Design review of the part built by this model. Coordinates are the model's own, in mm. Face numbers are marked on the shaded views. A direction names the side the tool comes from. Round coordinates to 2 decimals unless told otherwise and drop trailing zeros. Loops run counter-clockwise (first coordinate to the right, second up) from the corner with the lowest first, then second, coordinate; pieces in that order, holes last. Notation, with made-up numbers: (-16.75, 10) -> (-5.75, 10) arc R26 ccw to (-5.75, 32) -> close; hole circle Ø6 at (38, -12.75). An arc over 180 degrees is marked (long way). Write each question's results on one line, items separated by ' | '. Start each with the question number.
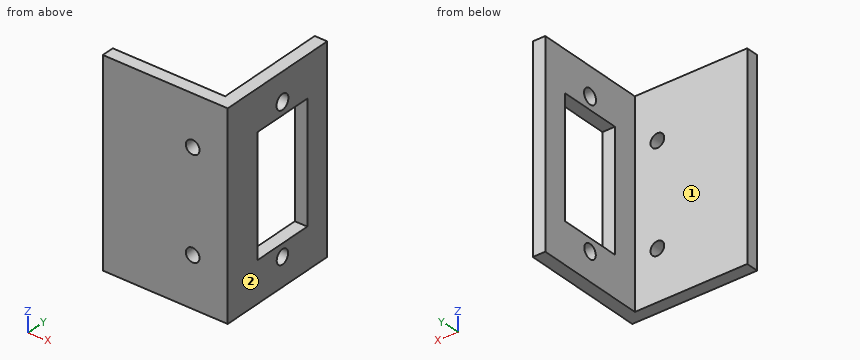
from build123d import *

# Parameters (mm, degrees)
EXTRUDE_1_DEPTH     = 16
SKETCH_4_R          = 1.15
SKETCH_4_R_2        = 1.2
SKETCH_4_W          = 19
SKETCH_4_H          = 10
CUT_EXTRUDE_1_DEPTH = 30
SKETCH_5_R          = 1.1
CUT_EXTRUDE_2_DEPTH = 30


with BuildPart() as part:
    # 草图2 → 凸台-拉伸1 (new body, symmetric)
    with BuildSketch(Plane.XY):
        Polygon((-20, 0), (0, 0), (0, 20), (-2, 20), (-2, 2), (-20, 2), align=None)
    extrude(amount=EXTRUDE_1_DEPTH, both=True)

    # 草图4 → 切除-拉伸1 (cut)
    with BuildSketch(Plane(origin=(0, 0, 0), x_dir=(0, 0, -1), z_dir=(1, 0, 0))):
        with Locations((11.5, 11)):
            Circle(SKETCH_4_R)
        with Locations((-11.5, 11)):
            Circle(SKETCH_4_R_2)
        with Locations((0, 11)):
            Rectangle(SKETCH_4_W, SKETCH_4_H)
    extrude(amount=-CUT_EXTRUDE_1_DEPTH, mode=Mode.SUBTRACT)

    # 草图5 → 切除-拉伸2 (cut)
    with BuildSketch(Plane(origin=(0, 2, 0), x_dir=(1, 0, 0), z_dir=(0, 1, 0))):
        with Locations((-5.609756098, 8)):
            Circle(SKETCH_5_R)
        with Locations((-5.609756098, -8)):
            Circle(SKETCH_5_R)
    extrude(amount=-CUT_EXTRUDE_2_DEPTH, mode=Mode.SUBTRACT)


solid = part.part
1) Insertion check: pin 1 (5.5 mm diameter, centred on x = -13.5, z = -4.5, fed in from +Y); pin 2 (5 mm diameter, centred on x = -17.5, z = 12, fed in from -Y); pin 3 (2 mm diameter, centred on y = 12.5, z = -9, fed in from -X). Each pin has a flat end and moves straight along its axis. Give the tip position at first contact, or say it passes through.
2) To check wall thickness, follow line 1 (X direction, y = 1.5, z = 8); line 2 (Y direction, x = -0.5, z = -11.5); line 3 (Y direction, x = -1, z = -2). State the ranges of each line that lie inside material, in increasing order. Write a range as from..to.
3) For the marked faces 1 and 2, list the 3-axis set-ups (+Z, -Z, +X, -X, +Y, -Y) from which the entire face can be reached by the end or side of a thin tool; tool diameter is ignored.
4) Take a section at A-A (z = -11.5). Write out the cut boundary in (x, y), plus the area to 3 significant figures.
5) Take a section at D-D (y = 11). Write out the cut boundary in (x, z), plus the area to 3 significant figures.
6) Take a section at C-C (z = -8). Write out the cut boundary in (x, y), plus the area to 3 significant figures.
7) Take a section at B-B (y = 14). Write out the cut boundary in (x, z).
Geometry check:
1) pin 1: stops at y = 2 | pin 2: stops at y = 0 | pin 3: stops at x = -2
2) line 1: x = -20..-6.71, -4.51..0 | line 2: y = 0..9.85, 12.15..20 | line 3: y = 0..6, 16..20
3) face 1: +Z, -Z, -X, +Y | face 2: +Z, -Z, +X, +Y, -Y
4) outline: (-20, 0) -> (0, 0) -> (0, 9.85) -> (-2, 9.85) -> (-2, 2) -> (-20, 2) -> close; (-2, 12.15) -> (0, 12.15) -> (0, 20) -> (-2, 20) -> close | area: 71.4 mm^2
5) outline: (-2, -16) -> (0, -16) -> (0, -12.65) -> (-2, -12.65) -> close; (-2, -10.35) -> (0, -10.35) -> (0, -9.5) -> (-2, -9.5) -> close; (-2, 9.5) -> (0, 9.5) -> (0, 10.3) -> (-2, 10.3) -> close; (-2, 12.7) -> (0, 12.7) -> (0, 16) -> (-2, 16) -> close | area: 16.6 mm^2
6) outline: (-20, 0) -> (-6.71, 0) -> (-6.71, 2) -> (-20, 2) -> close; (-4.51, 0) -> (0, 0) -> (0, 6) -> (-2, 6) -> (-2, 2) -> (-4.51, 2) -> close; (-2, 16) -> (0, 16) -> (0, 20) -> (-2, 20) -> close | area: 51.6 mm^2
7) outline: (-2, -16) -> (0, -16) -> (0, -9.5) -> (-2, -9.5) -> close; (-2, 9.5) -> (0, 9.5) -> (0, 16) -> (-2, 16) -> close
